Design review of the part built by this model. Coordinates are the model's own, in mm. A direction names the side the tool comes from. Round coordinates to 2 decimals unless told otherwise and drop trailing zeros. Order: outer loops, then holes, each group sorted by start corner. A loop starts at its lowest first (then second) coordinate and runs counter-clockwise, first axis right, second up. Notation, with made-up numbers: (72, -14) - (103, -14) arc R19 ccw to (103, -5) - close; hole circle Ø6 at (30, 61). An arc over 180 degrees is marked (long way). Write item = value, one per line.
from build123d import *

# Parameters (mm, degrees)
SKETCH1_R           = 20
BOSS_EXTRUDE1_DEPTH = 12.7
SKETCH2_R           = 1.5875
CUT_EXTRUDE1_DEPTH  = 88.081184849
SKETCH4_W           = 20.078494948
SKETCH4_H           = 48.78095735
SKETCH4_W_2         = 48.420880553
SKETCH4_H_2         = 19.195923741
CUT_EXTRUDE2_DEPTH  = 26.162
SKETCH5_R           = 3.175
CUT_EXTRUDE3_DEPTH  = 11.43
SKETCH6_R           = 3.175
CUT_EXTRUDE4_DEPTH  = 11.43


with BuildPart() as part:
    # Sketch1 → Boss-Extrude1 (new body)
    with BuildSketch(Plane(origin=(0, 0, 0), x_dir=(0, 0, -1), z_dir=(1, 0, 0))):
        with BuildLine():
            Line((0, 31.882172919), (31.882172919, 31.882172919))
            Line((31.882172919, 31.882172919), (60.87463474, 31.882172919))
            Line((60.87463474, 31.882172919), (60.87463474, -60.96))
            Line((60.87463474, -60.96), (-31.882172919, -60.96))
            Line((-31.882172919, -60.96), (-31.882172919, 0))
            ThreePointArc((-31.882172919, 0), (-22.54410067, 22.54410067), (0, 31.882172919))
        make_face()
        Circle(SKETCH1_R, mode=Mode.SUBTRACT)
    extrude(amount=BOSS_EXTRUDE1_DEPTH)

    # Sketch2 → Cut-Extrude1 (cut, through all)
    with BuildSketch(Plane(origin=(0, 0, 0), x_dir=(1, 0, 0), z_dir=(0, 1, 0))):
        with Locations(Location((6.35, 0, 0), (0, 0, 90))):
            Circle(SKETCH2_R)
    extrude(amount=CUT_EXTRUDE1_DEPTH, mode=Mode.SUBTRACT)

    # Sketch4 → Cut-Extrude2 (cut)
    with BuildSketch(Plane.ZY):
        with Locations((-43.731401429, -0.427222634)):
            Rectangle(SKETCH4_W, SKETCH4_H)
        with Locations((-0.75610861, -42.339905849)):
            Rectangle(SKETCH4_W_2, SKETCH4_H_2)
        with Locations((-43.731401429, -42.339905849)):
            Rectangle(SKETCH4_W, SKETCH4_H_2)
    extrude(amount=-CUT_EXTRUDE2_DEPTH, mode=Mode.SUBTRACT)

    # Sketch5 → Cut-Extrude3 (cut)
    with BuildSketch(Plane(origin=(0, 0, -60.87463474), x_dir=(-1, 0, 0), z_dir=(0, 0, -1))):
        with Locations((-6.35, 16.187024645)):
            Circle(SKETCH5_R)
        with Locations((-6.35, -44.788648077)):
            Circle(SKETCH5_R)
    extrude(amount=-CUT_EXTRUDE3_DEPTH, mode=Mode.SUBTRACT)

    # Sketch6 → Cut-Extrude4 (cut)
    with BuildSketch(Plane.XZ.offset(60.96)):
        with Locations(Location((6.35, 15.24, 0), (0, 0, 270))):
            Circle(SKETCH6_R)
        with Locations(Location((6.35, -45.41055385, 0), (0, 0, 270))):
            Circle(SKETCH6_R)
    extrude(amount=-CUT_EXTRUDE4_DEPTH, mode=Mode.SUBTRACT)


solid = part.part
1) Clearance check with flat-ended pins moving along their axes: pin 1 Ø5 at (x, y) = (6.35, 16.19) entering from -Z; pin 2 Ø4 at (x, z) = (6.35, 15.24) entering from +Y; pin 3 Ø4 at (x, z) = (6.35, -45.41) entering from -Y. State where each tip first meets the part, or that it passes through.
Findings:
pin_1 = -33.69
pin_2 = 29
pin_3 = -32.74
2) We need section D-D on z = -21.5. Write out the cut boundary in (x, y).
Findings:
outline = (0, -60.96) - (12.7, -60.96) - (12.7, -51.94) - (0, -51.94) - close; (0, -32.74) - (12.7, -32.74) - (12.7, 31.88) - (0, 31.88) - close
3) To check wall thickness, follow L1, parallel to Z at x = 6.25, y = -57; L2, parallel to Y at x = 6.35, z = -55.75; L3, parallel to X at y = -57.25, z = 15.24 (3 decimals). State the ranges of each line that lie inside material, in increasing order. Write a range as from..to.
Findings:
L1 = -60.87..-48.58, -42.24..12.07, 18.41..31.88
L2 = -60.96..-47.96, -41.61..13.01, 19.36..31.88
L3 = 0..3.175, 9.525..12.7
4) The part is to be moulded in two halves that separate along X. For faces 1 (the flat face through (12.7, -14, -15)), 2 (the flat face through (0, -14, -15)), 3 (the flat face through (6, -51.938, -42)), 4 (the cylindrical face through (7.76, 25.82, -0.73)), say which applies: released by +X, released by -X, zero draft, split by the parting line, or undercut.
Findings:
face_1 = released by +X
face_2 = released by -X
face_3 = zero draft
face_4 = undercut
5) We need section C-C on y = 5.5. Write out the cut boundary in (x, z), and give its area (3 significant figures).
Findings:
outline = (0, -60.87) - (12.7, -60.87) - (12.7, -53.77) - (0, -53.77) - close; (0, -33.69) - (12.7, -33.69) - (12.7, -19.23) - (0, -19.23) - close; (0, 19.23) - (12.7, 19.23) - (12.7, 31.4) - (0, 31.4) - close
area = 429 mm^2
6) We need section B-B on z = -40. Write out the cut boundary in (x, y), and give its area (3 significant figures).
Findings:
outline = (0, -60.96) - (12.7, -60.96) - (12.7, -51.94) - (0, -51.94) - close; (0, -32.74) - (12.7, -32.74) - (12.7, -24.82) - (0, -24.82) - close; (0, 23.96) - (12.7, 23.96) - (12.7, 31.88) - (0, 31.88) - close
area = 316 mm^2
7) We need section A-A on x = 1.75. Write out the cut boundary in (y, z), and give its area (3 significant figures).
Findings:
outline = (-60.96, -60.87) - (31.88, -60.87) - (31.88, 0) arc R31.88 ccw to (0, 31.88) - (-60.96, 31.88) - close; hole (-51.94, -53.77) - (-32.74, -53.77) - (-32.74, -33.69) - (-51.94, -33.69) - close; hole (-51.94, -24.97) - (-32.74, -24.97) - (-32.74, 23.45) - (-51.94, 23.45) - close; hole (-24.82, -53.77) - (23.96, -53.77) - (23.96, -33.69) - (-24.82, -33.69) - close; hole circle Ø40 at (0, 0)
area = 4,840 mm^2
8) For faces 5 (the flat face through (6, -40, -53.771)), 6 (the flat face through (6, 31.882, -30)), 7 (the cylindrical face through (6.76, -41.64, -57.37)), list the 3-axis set-ups (+Z, -Z, +X, -X, +Y, -Y) from which the entire face can be reached by the end or side of a thin tool; tool diameter is ignored.
Findings:
face_5 = +X, -X
face_6 = +Z, -Z, +X, -X, +Y
face_7 = -Z
